from build123d import *

# Parameters (mm, degrees)
F0_R          = 52.3875
F0_R_2        = 50.8
F1_DEPTH      = 101.6
F5_R          = 26.9875
F5_R_2        = 25.4
F6_DEPTH      = 50.8
F6_DEPTH_BACK = 50.8
F7_DEPTH      = 105.8050688415
F7_DEPTH_BACK = 4.2050688415
F8_DEPTH      = 50.8
F8_DEPTH_BACK = 77.7885001414


with BuildPart() as f1:
    # F0 (on Top) → F1 (new body)
    with BuildSketch(Plane.XY):
        Circle(F0_R)
        Circle(F0_R_2, mode=Mode.SUBTRACT)
    extrude(amount=F1_DEPTH)

    # F5 (on line) → F6 (join, two sides)
    with BuildSketch(Plane(origin=(51.59375, 0, 51.59375), x_dir=(0.7071067812, 0, -0.7071067812), z_dir=(0.7071067812, 0, 0.7071067812))) as f6_sk:
        with Locations((1.1225320151, 0)):
            Circle(F5_R)
        with Locations((1.1225320151, 0)):
            Circle(F5_R_2, mode=Mode.SUBTRACT)
    extrude(amount=F6_DEPTH)
    extrude(f6_sk.sketch, amount=-F6_DEPTH_BACK)

    # F0 (on Top) → F7 (cut, two sides)
    with BuildSketch(Plane.XY) as f7_sk:
        Circle(F0_R_2)
    extrude(amount=F7_DEPTH, mode=Mode.SUBTRACT)
    extrude(f7_sk.sketch, amount=-F7_DEPTH_BACK, mode=Mode.SUBTRACT)

    # F5 (on line) → F8 (cut, two sides)
    with BuildSketch(Plane(origin=(51.59375, 0, 51.59375), x_dir=(0.7071067812, 0, -0.7071067812), z_dir=(0.7071067812, 0, 0.7071067812))) as f8_sk:
        with Locations((1.1225320151, 0)):
            Circle(F5_R_2)
    extrude(amount=-F8_DEPTH, mode=Mode.SUBTRACT)
    extrude(f8_sk.sketch, amount=F8_DEPTH_BACK, mode=Mode.SUBTRACT)


solid = f1.part
Read the model definition and answer for the solid it produces. Units are mm, in the model's axes. A direction names the side the tool comes from. Coordinates: 2 decimals unless noted, no trailing zeros. Order: outer loops, then holes, each group sorted by start corner. A loop starts at its lowest first (then second) coordinate and runs counter-clockwise, first axis right, second up. Notation, with made-up numbers: (-6.75, 18.5) - (0.25, 18.5) arc R29 ccw to (0.25, 46.5) - close; hole circle Ø7 at (-0.5, 71.5). An arc over 180 degrees is marked (long way). Use one line per item in the form item = value.
(1) Section D-D, the plane y = -19 is taken. Give the vertices of the cut face in (x, z), then the cut area to 3 significant figures.
Computed values:
outline = (-48.82, 0) - (-47.11, 0) - (-47.11, 101.6) - (-48.82, 101.6) - close; (47.11, 0) - (48.82, 0) - (48.82, 20.13) - (101.86, 73.17) - (100.23, 74.8) - (47.11, 21.69) - close; (47.11, 69.37) - (76.39, 98.64) - (74.76, 100.27) - (48.82, 74.34) - (48.82, 101.6) - (47.11, 101.6) - close
area = 523 mm²
(2) Section A-A, the plane y = -3 is taken. Give the vertices of the cut face in (x, z), then the cut area to 3 significant figures.
Computed values:
outline = (-52.3, 0) - (-50.71, 0) - (-50.71, 101.6) - (-52.3, 101.6) - close; (50.71, 0) - (52.3, 0) - (52.3, 12.78) - (107.27, 67.76) - (106.14, 68.89) - (50.71, 13.45) - close; (50.71, 84.79) - (70.47, 104.56) - (69.34, 105.69) - (52.3, 88.64) - (52.3, 101.6) - (50.71, 101.6) - close
area = 372 mm²
(3) Section B-B, the plane x = -10.5 is taken. Give the vertices of the cut face in (y, z).
Computed values:
outline = (-51.32, 0) - (-49.7, 0) - (-49.7, 101.6) - (-51.32, 101.6) - close; (49.7, 0) - (51.32, 0) - (51.32, 101.6) - (49.7, 101.6) - close
(4) Section C-C, the plane x = 30.5 is taken. Give the vertices of the cut face in (y, z) (3 decimals).
Computed values:
outline = (-42.593, 0) - (-40.625, 0) - (-40.625, 101.6) - (-42.593, 101.6) - close; (40.625, 0) - (42.593, 0) - (42.593, 101.6) - (40.625, 101.6) - close
(5) Given pin 1 Ø12 at (x, z) = (12, 79) entering from -Y; pin 2 Ø1 at (x, z) = (12, 50.5) entering from +Y; pin 3 Ø12 at (x, z) = (-8.5, 48.5) entering from +Y, each flat-ended and moving along its own axis, determine where each tip first touches the part or whether it passes through.
Computed values:
pin_1 = -52.04
pin_2 = 51.11
pin_3 = 52.33
(6) Straight lines are drawn through the part: L1, parallel to Y at x = 1, z = 6; L2, parallel to X at y = -22, z = 13; L3, parallel to Y at x = -10, z = 84. For each, find the intervals that lie inside material, in ascending order.
Computed values:
L1 = -52.38 to -50.79, 50.79 to 52.38
L2 = -47.54 to -45.79, 45.79 to 47.54
L3 = -51.42 to -49.81, 49.81 to 51.42
(7) Which of the six approach directions +Z, -Z, +X, -X, +Y, -Y give full straight-line access (tool end or side, diameter ignored) to faces 1 (the face through (105.18, -9.87, 69.85)), 2 (the face through (-51, 4, 101.6))?
Computed values:
face_1 = +Z, +X, +Y, -Y
face_2 = +Z, -X, +Y, -Y
